Work out the finished part from the listing and answer in its coordinate system (mm). A direction names the side the tool comes from. Give positions to 0.01 mm unless a question says otherwise; leave off trailing zeros. Loops run counter-clockwise (first coordinate to the right, second up) from the corner with the lowest first, then second, coordinate; pieces in that order, holes last. Notation, with made-up numbers: (10, 47) - (27, 47) arc R24 cw to (27, 76) - close; hole circle Ø4 at (25, 26). An arc over 180 degrees is marked (long way). One line per question, with ' | ' between items. Start each with the question number.
1. Which of the six approach directions +Z, -Z, +X, -X, +Y, -Y give full straight-line access (tool end or side, diameter ignored) to faces 4 (the face through (79, 2, 127)), 5 (the face through (7.61, 3.52, 6.69)), 6 (the face through (69, 3, 16.51))?
2. Section B-B (x = 5.08) is taken. Determine the outline of the cut face in (y, z).
3. For a pull along X with two mould halves and no side action, classify faces 1 (the face through (53, 0, 63)), 2 (the face through (0, 2, 34)), 3 (the face through (69, 3, 10.16)) as released by +X, released by -X, zero draft, split by the parting line, or undercut.
4. Find the intervals of material crossed by line 1 (X direction, y = 1.3, z = 5.08); line 2 (X direction, y = 4.15, z = 5.08); line 3 (Z direction, x = 64.5, y = 0.7), in increasing order.
5. Section C-C (z = 5.08) is taken. Determine the outline of the cut face in (x, y).
6. Section D-D (y = 3.8) is taken. Give the number of separate pieces and of enclosed holes in the cut face, plus the area to 3 significant figures.
7. Each of these flat-tipped pins is pushed along its axis until it touches: pin 1 (3 mm diameter, centred on x = 98, z = 5, fed in from +Y); pin 2 (2 mm diameter, centred on x = 27, y = 3, fed in from +Z). Where does it stop, or does it pass through?
8. Section A-A (z = 63.08) is taken. Determine the outline of the cut face in (x, y).
from build123d import *

# Parameters (mm, degrees)
BOSS_EXTRUDE1_DEPTH   = 5
F_4_0MM_DOWEL_HOLE1_D = 3.3
SKETCH4_W             = 12.7
SKETCH4_H             = 6.35
CUT_EXTRUDE1_DEPTH    = 5
FILLET1_R             = 2
SKETCH5_R             = 3
CUT_EXTRUDE2_DEPTH    = 3


with BuildPart() as part:
    # Sketch1 → Boss-Extrude1 (new body)
    with BuildSketch(Plane(origin=(0, 0, 0), x_dir=(1, 0, 0), z_dir=(0, 1, 0))):
        Polygon((0, 0), (104.14, 0), (104.140084457, -68.379681711), (104.140084457, -126.999681711), (52.560084457, -126.999681711), (0, -67.34), align=None)
    extrude(amount=BOSS_EXTRUDE1_DEPTH)

    # Ø4.0mm Dowel Hole1 (through all)
    with Locations(Plane(origin=(5.08, 5, 5.08), x_dir=(0, 0, 1), z_dir=(0, 1, 0))):
        with Locations((0, 0), (0, 47.95), (0, 93.980006274), (116.839681711, 93.980084457), (116.839681711, 50.770084457), (89.156056724, 25.385630403), (58, 0)):
            Hole(F_4_0MM_DOWEL_HOLE1_D / 2)

    # Sketch4 → Cut-Extrude1 (cut)
    with BuildSketch(Plane(origin=(0, 5, 0), x_dir=(1, 0, 0), z_dir=(0, 1, 0))):
        with Locations((69, -13.335)):
            Rectangle(SKETCH4_W, SKETCH4_H)
    extrude(amount=-CUT_EXTRUDE1_DEPTH, mode=Mode.SUBTRACT)

    # Fillet1
    fillet1_edges = [part.edges().sort_by_distance(p)[0] for p in [
        (62.65, 2.5, 10.16),
        (62.65, 2.5, 16.51),
        (75.35, 2.5, 16.51),
        (75.35, 2.5, 10.16),
    ]]
    fillet(fillet1_edges, radius=FILLET1_R)

    # Sketch5 → Cut-Extrude2 (cut)
    with BuildSketch(Plane(origin=(0, 5, 0), x_dir=(1, 0, 0), z_dir=(0, 1, 0))):
        with Locations(Location((55.850084457, -121.919681711, 0), (0, 0, 270))):
            Circle(SKETCH5_R)
        with Locations(Location((99.060084457, -121.919681711, 0), (0, 0, 270))):
            Circle(SKETCH5_R)
        with Locations(Location((30.465630403, -94.236056724, 0), (0, 0, 270))):
            Circle(SKETCH5_R)
        with Locations(Location((5.08, -63.08, 0), (0, 0, 270))):
            Circle(SKETCH5_R)
        with Locations(Location((5.08, -5.08, 0), (0, 0, 270))):
            Circle(SKETCH5_R)
        with Locations(Location((53.03, -5.08, 0), (0, 0, 270))):
            Circle(SKETCH5_R)
        with Locations(Location((99.060006274, -5.08, 0), (0, 0, 270))):
            Circle(SKETCH5_R)
    extrude(amount=-CUT_EXTRUDE2_DEPTH, mode=Mode.SUBTRACT)


solid = part.part
Conclusion:
1) face 4: +Z, +X, -X, +Y, -Y | face 5: +Y | face 6: +Y, -Y
2) outline: (0, 0) - (5, 0) - (5, 2.08) - (2, 2.08) - (2, 3.43) - (0, 3.43) - close; (0, 6.73) - (2, 6.73) - (2, 8.08) - (5, 8.08) - (5, 60.08) - (2, 60.08) - (2, 61.43) - (0, 61.43) - close; (0, 64.73) - (2, 64.73) - (2, 66.08) - (5, 66.08) - (5, 73.11) - (0, 73.11) - close
3) face 1: zero draft | face 2: released by -X | face 3: undercut
4) line 1: 0 to 3.43, 6.73 to 51.38, 54.68 to 97.41, 100.71 to 104.14 | line 2: 0 to 2.08, 8.08 to 50.03, 56.03 to 96.06, 102.06 to 104.14 | line 3: 0 to 10.17, 16.5 to 127
5) outline: (0, 0) - (3.43, 0) - (3.43, 2) - (2.08, 2) - (2.08, 5) - (0, 5) - close; (6.73, 0) - (51.38, 0) - (51.38, 2) - (50.03, 2) - (50.03, 5) - (8.08, 5) - (8.08, 2) - (6.73, 2) - close; (54.68, 0) - (97.41, 0) - (97.41, 2) - (96.06, 2) - (96.06, 5) - (56.03, 5) - (56.03, 2) - (54.68, 2) - close; (100.71, 0) - (104.14, 0) - (104.14, 5) - (102.06, 5) - (102.06, 2) - (100.71, 2) - close
6) separate pieces: 1 | enclosed holes: 8 | area: 11,400 mm²
7) pin 1: y = 2 | pin 2: z = 99.12
8) outline: (0, 0) - (3.43, 0) - (3.43, 2) - (2.08, 2) - (2.08, 5) - (0, 5) - close; (6.73, 0) - (104.14, 0) - (104.14, 5) - (8.08, 5) - (8.08, 2) - (6.73, 2) - close
